Can you work these out from the model? Positions are in its coordinate system, mm. Round coordinates to 2 decimals unless told otherwise and drop trailing zeros. Write each loop counter-clockwise with the first axis right and the second up, starting at its lowest first coordinate (ties: lowest second). Pieces come first, ordered by that corner, then holes. Notation, with made-up numbers: M -25,34 L 28,34 A20 cw 28,58 Z; hole C 20,-12.5 d5. An arc over 180 degrees is marked long. Answer as a JSON object with one key per item and string values. Group by question number.
1) If we mould it in two halves opening along Z, with no side actions, what happens to faces 1 (the flat face through (19, 3, 0)), 2 (the cylindrical face through (20.004, 3.219, 90.955)), 3 (the flat face through (0, 3, 56))? For each: +Z half, -Z half, draft (parallel to the pull), parting line (faces both ways), or undercut.
2) Suppose I cut it at C-C, the plane y = 1.5. Write out the boundary of the cut face in (x, z), and give its area (3 significant figures).
3) Suppose I cut it at D-D, the plane z = 21.5. Write out the boundary of the cut face in (x, y), and give its area (3 significant figures).
4) Please list where these lines run through material, in increasing order: L1, parallel to Z at x = 19.05, y = 4.25; L2, parallel to Z at x = 15, y = 3; L3, parallel to X at y = 5.25, z = 97.5. Write a range as [from, to].
5) Suppose I cut it at B-B, the plane z = 95.25. Write out the boundary of the cut face in (x, y), and give its area (3 significant figures).
6) I'm going to push flat-ended pins straight in: pin 1 Ø10 at (x, z) = (33, 66.5) entering from -Y; pin 2 Ø7 at (x, z) = (19.05, 19.05) entering from +Y. Where does each tip first touch, or does it pass through?
7) Suppose I cut it at A-A, the plane x = 19.05. Write out the boundary of the cut face in (y, z), and give its area (3 significant figures).
from build123d import *

# Parameters (mm, degrees)
F0_W     = 38.1
F0_H     = 114.3
F1_DEPTH = 6.35
F2_D     = 8.8


# Not quite as in the source:
# - a length typed as a fraction of an inch, garbled in the dataset ("3 / 203.2 mm" for 3/8 in), is restored
# - a feature names something its author has since deleted; it is built from what else it names


with BuildPart() as f1:
    # F0 (on Front) → F1 (new body)
    with BuildSketch(Plane.XZ):
        with Locations((19.05, 57.15)):
            Rectangle(F0_W, F0_H)
    extrude(amount=-F1_DEPTH)

    # F2 (through all)
    with Locations(Plane.XZ):
        with Locations((19.05, 95.25), (19.05, 57.15), (19.05, 19.05)):
            Hole(F2_D / 2)


solid = f1.part
Results:
{
 "1": {"face 1": "-Z half", "face 2": "undercut", "face 3": "draft"},
 "2": {"outline": "M 0,0 L 38.1,0 L 38.1,114.3 L 0,114.3 Z; hole C 19.05,19.05 d8.8; hole C 19.05,57.15 d8.8; hole C 19.05,95.25 d8.8", "area": "4,170 mm^2"},
 "3": {"outline": "M 0,0 L 15.4,0 L 15.4,6.35 L 0,6.35 Z; M 22.7,0 L 38.1,0 L 38.1,6.35 L 22.7,6.35 Z", "area": "196 mm^2"},
 "4": {"L1": "[0, 14.65], [23.45, 52.75], [61.55, 90.85], [99.65, 114.3]", "L2": "[0, 17.33], [20.77, 55.43], [58.87, 93.53], [96.97, 114.3]", "L3": "[0, 15.27], [22.83, 38.1]"},
 "5": {"outline": "M 0,0 L 14.65,0 L 14.65,6.35 L 0,6.35 Z; M 23.45,0 L 38.1,0 L 38.1,6.35 L 23.45,6.35 Z", "area": "186 mm^2"},
 "6": {"pin 1": "y = 0", "pin 2": "through"},
 "7": {"outline": "M 0,0 L 6.35,0 L 6.35,14.65 L 0,14.65 Z; M 0,23.45 L 6.35,23.45 L 6.35,52.75 L 0,52.75 Z; M 0,61.55 L 6.35,61.55 L 6.35,90.85 L 0,90.85 Z; M 0,99.65 L 6.35,99.65 L 6.35,114.3 L 0,114.3 Z", "area": "558 mm^2"}
}
